Design review of the part built by this model. Coordinates are the model's own, in mm. Face numbers are marked on the shaded views. A direction names the side the tool comes from. Round coordinates to 2 decimals unless told otherwise and drop trailing zeros. Order: outer loops, then holes, each group sorted by start corner. A loop starts at its lowest first (then second) coordinate and runs counter-clockwise, first axis right, second up. Notation, with made-up numbers: (5.5, 42.5) - (25.5, 42.5) arc R14 ccw to (25.5, 64.5) - close; hole circle Ø6 at (5, 49.5). An arc over 180 degrees is marked (long way). Use CSV: the item, a comma, the result in double quotes.
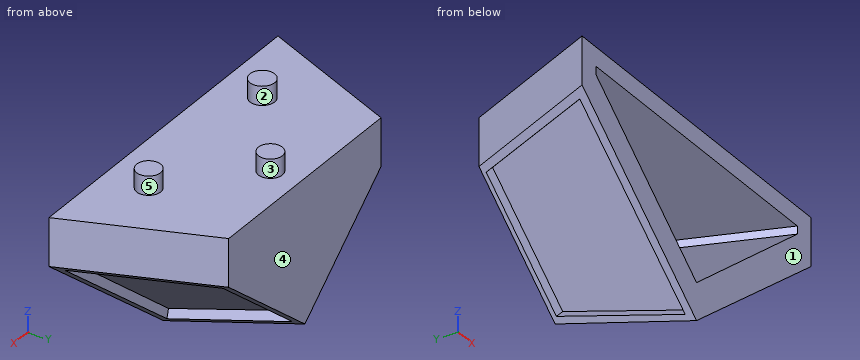
from build123d import *

# Parameters (mm, degrees)
SKETCH8_R           = 1.614382249
SKETCH8_R_2         = 1.666459096
BOSS_EXTRUDE1_DEPTH = 2.54
CUT_EXTRUDE1_DEPTH  = 1.27
CUT_EXTRUDE3_DEPTH  = 1.27


with BuildPart() as part:
    # Sketch7 → Loft1 section 0
    with BuildSketch(Plane(origin=(0, 19.05, 0), x_dir=(1, 0, 0), z_dir=(0, 1, 0))):
        with BuildLine():
            Line((2.329927564, -19.831697395), (-28.030874095, -19.831697395))
            Line((-28.030874095, -19.831697395), (-28.030874095, -13.401990643))
            Line((-28.030874095, -13.401990643), (-12.850473266, -0.591086342))
            Line((-12.850473266, -0.591086342), (2.329927564, -13.401990643))
            Line((2.329927564, -13.401990643), (2.329927564, -19.831697395))
        make_face()
    # Sketch1 → Loft1 section 1
    with BuildSketch(Plane(origin=(0, 0, 0), x_dir=(1, 0, 0), z_dir=(0, 1, 0))):
        with BuildLine():
            Line((-35.720948922, -19.831697395), (9.915848697, -19.831697395))
            Line((9.915848697, -19.831697395), (9.915848697, -13.380422339))
            Line((9.915848697, -13.380422339), (-12.902550112, 5.734466717))
            Line((-12.902550112, 5.734466717), (-35.720948922, -13.380422339))
            Line((-35.720948922, -13.380422339), (-35.720948922, -19.831697395))
        make_face()
    loft()

    # Sketch8 → Boss-Extrude1 (add)
    with BuildSketch(Plane.XY.offset(19.831697395)):
        with Locations((-11.991205294, 14.993068909)):
            Circle(SKETCH8_R)
        with Locations((-1.47168225, 5.723390187)):
            Circle(SKETCH8_R)
        with Locations((-24.125110588, 5.723390187)):
            Circle(SKETCH8_R_2)
    extrude(amount=BOSS_EXTRUDE1_DEPTH)

    # Sketch10 → Cut-Extrude1 (cut)
    with BuildSketch(Plane(origin=(-2.316668622, -0.925631174, 2.745158144), x_dir=(-0.7809926786782739, 0.19954822136443426, -0.5918031287524808), z_dir=(0.6245401795328581, 0.2495367072226862, -0.7400547249342612))):
        Polygon((-5.325710862, 21.043562966), (-13.739013708, 5.028281727), (12.35928027, -0.480841902), (12.35928027, 17.367594826), align=None)
    extrude(amount=-CUT_EXTRUDE1_DEPTH, mode=Mode.SUBTRACT)

    # Sketch14 → Cut-Extrude3 (cut)
    with BuildSketch(Plane(origin=(-7.735349681, 3.132971893, -9.166074927), x_dir=(-0.7814202870497631, -0.2018218164714577, 0.5904661627758421), z_dir=(-0.6240050760907847, 0.25273458150056255, -0.7394206491075764))):
        Polygon((34.101698791, 5.249617187), (25.261874217, 21.574256729), (7.477459861, 17.716608027), (7.477459861, -0.525493463), align=None)
    extrude(amount=-CUT_EXTRUDE3_DEPTH, mode=Mode.SUBTRACT)

    # Shell1: read off the stored shape, not the designer's step
    # Shell1: loft between two sections, ruled curve by curve
    shell1_from = [
        Edge.make_line((-32.981801445, 0, 17.291697395), (-32.981801445, 0, 16.221508901)),
        Edge.make_line((7.181869263, 0, 16.221455471), (7.181869263, 0, 17.291697395)),
        Edge.make_line((-32.981801445, 0, 17.291697395), (7.181869263, 0, 17.291697395)),
        Edge.make_line((7.181869263, 0, 16.221455471), (-12.899934435, 0, -0.725795677)),
        Edge.make_line((-32.981801445, 0, 16.221508901), (-12.899934435, 0, -0.725795677)),
    ]
    shell1_to = [
        Edge.make_line((-26.317069927, 16.51, 17.291697395), (-26.317069927, 16.51, 16.240201431)),
        Edge.make_line((0.607404281, 16.51, 16.240148002), (0.607404281, 16.51, 17.291697395)),
        Edge.make_line((-26.317069927, 16.51, 17.291697395), (0.607404281, 16.51, 17.291697395)),
        Edge.make_line((0.607404281, 16.51, 16.240148002), (-12.854801168, 16.51, 4.879247349)),
        Edge.make_line((-26.317069927, 16.51, 16.240201431), (-12.854801168, 16.51, 4.879247349)),
    ]
    shell1 = Solid(Shell([*[Face.make_surface_from_curves(shell1_from[k], shell1_to[k]) for k in range(5)], Face(Wire(shell1_from)), Face(Wire(shell1_to))]))
    add(shell1, mode=Mode.SUBTRACT)


solid = part.part
1) The part is to be moulded in two halves that separate along X. For the marked faces 3, 4 and 5, say which applies: +X half, -X half, draft (parallel to the pull), parting line (faces both ways), or undercut.
Data:
face 3,"parting line"
face 4,"draft"
face 5,"undercut"
2) To check wall thickness, follow L1, parallel to X at y = 10.5, z = 13; L2, parallel to Y at x = -15, z = 10.75; L3, parallel to X at y = 6.25, z = 13. State the ranges of each line that lie inside material, in increasing order. Write a range as from..to.
Data:
L1,"x = -31.02..-30.37, -28.98..-24.91, -0.83..3.24, 4.32..5.27"
L2,"y = 16.51..19.05"
L3,"x = -32.74..-32.06, -30.7..-26.63, 0.87..4.93, 5.94..6.97"
3) For the marked faces 1 and 2, list the 3-axis set-ups (+Z, -Z, +X, -X, +Y, -Y) from which the entire face can be reached by the end or side of a thin tool; tool diameter is ignored.
Data:
face 1,"+Z, -Z, +X, -X, -Y"
face 2,"+Z"
4) Insertion check: pin 1 Ø3.5 at (x, z) = (-17.5, 12) entering from -Y; pin 2 Ø1 at (y, z) = (8.5, 15.5) entering from -X; pin 3 Ø1 at (x, y) = (-29, 14.5) entering from +Z. Each pin has a flat end and moves straight along its axis. Give the tip position at first contact, or say it passes through.
Data:
pin 1,"stops at y = 16.51"
pin 2,"stops at x = -32.49"
pin 3,"stops at z = 19.83"
5) We need section A-A (z = 20.5). Give the boundary of the cut face in (x, y).
Data:
outline,"circle Ø3.33 at (-24.13, 5.72); circle Ø3.23 at (-11.99, 14.99); circle Ø3.23 at (-1.47, 5.72)"
